Source: CAD feature listing. Evaluate the final solid. Frame: model axes, mm. A direction names the side the tool comes from. Round coordinates to 2 decimals unless told otherwise and drop trailing zeros. Loops run counter-clockwise (first coordinate to the right, second up) from the corner with the lowest first, then second, coordinate; pieces in that order, holes last. Notation, with made-up numbers: M 82.25,16.5 L 117.25,16.5 A23 ccw 117.25,34.5 Z; hole C -13.5,30 d4. An arc over 180 degrees is marked long. Write each question's results on one line, items separated by ' | '. Start each with the question number.
1. Set-up query: faces 1 (the flat face through (6, 2, -1)), 2 (the flat face through (11, 31, 0)), 3 (the flat face through (5, 18, -6.5)), 4 (the cylindrical face through (78.986, 8.474, -7.648)), 5 (the cylindrical face through (12.4, 25.27, 14.01)). Return all of +Z, -Z, +X, -X, +Y, -Y with unobstructed straight access to the full face (end or side cutting, diameter ignored); none if empty.
2. Section B-B on y = 18.5. Output: boundary loops of the cut face in (x, z), and give its area (3 significant figures).
3. Contact query for flat-ended pins moving along their axis: pin 1 Ø2 at (x, z) = (9.5, 0.5) entering from +Y; pin 2 Ø5 at (x, z) = (15, 0) entering from -Y; pin 3 Ø9 at (x, z) = (55.5, 0) entering from +Y; pin 4 Ø13 at (y, z) = (22, -2.5) entering from +X. Output: stop coordinate, or through.
4. Ray query, line 1 (Y direction, x = 3.75, z = 9); line 2 (Z direction, x = 8, y = 20.5); line 3 (Z direction, x = 12.5, y = 23.5). Return the intervals inside material, ascending.
5. Section D-D on z = 0. Give the number of separate pieces and of enclosed holes in the cut face, and give its area (3 significant figures).
6. Draft query along Z for faces 6 (the cylindrical face through (40.53, 0.57, 14.4)), 7 (the cylindrical face through (7, 32, 6)), 8 (the cylindrical face through (11.43, 34.4, 14.01)). Return one class per face: released by +Z, released by -Z, zero draft, split by the parting line, or undercut.
7. Section C-C on x = 44. Output: boundary loops of the cut face in (y, z).
8. Section A-A on x = 70. Output: boundary loops of the cut face in (y, z), and give its area (3 significant figures).
from build123d import *

# Parameters (mm, degrees)
BOSS_EXTRUDE1_DEPTH = 15
FILLET2_R           = 10
FILLET3_R           = 2
FILLET4_R           = 2
SHELL1_START        = 2
SHELL1_OUTLINE_W    = 33
SHELL1_OUTLINE_H    = 26
SHELL1_DEPTH        = 76
SKETCH2_R           = 2
CUT_EXTRUDE1_DEPTH  = 88.82938005
BOSS_EXTRUDE2_START = 6
SKETCH3_R           = 4
SKETCH3_R_2         = 2
BOSS_EXTRUDE2_DEPTH = 6
SKETCH4_W           = 26
SKETCH4_H           = 31
BOSS_EXTRUDE3_DEPTH = 10
SKETCH5_W           = 8
SKETCH5_H           = 8
CUT_EXTRUDE2_DEPTH  = 31
SKETCH6_W           = 8
SKETCH6_H           = 2
CUT_EXTRUDE3_DEPTH  = 6
FILLET5_R           = 5
FILLET6_R           = 2
SKETCH7_R           = 2
CUT_EXTRUDE4_DEPTH  = 89.600225733
CUT_EXTRUDE6_DEPTH  = 10


# Read off the part's stored shape, not the designer's step: Shell1
# Some blends are built 0.0001 mm under size
with BuildPart() as part:
    # Sketch1 → Boss-Extrude1 (new, symmetric)
    with BuildSketch(Plane.XY):
        with BuildLine():
            Line((0, 35), (0, 0))
            Line((0, 0), (80, 0))
            Line((80, 0), (80, 10))
            Line((80, 10), (60, 10))
            Line((60, 10), (13.403450014, 24.561421871))
            ThreePointArc((13.403450014, 24.561421871), (12.388618609, 25.28570887), (12, 26.470381827))
            Line((12, 26.470381827), (12, 33))
            ThreePointArc((12, 33), (11.414213562, 34.414213562), (10, 35))
            Line((10, 35), (0, 35))
        make_face()
    extrude(amount=BOSS_EXTRUDE1_DEPTH, both=True)

    # Fillet2
    fillet2_edges = [part.edges().sort_by_distance(p)[0] for p in [
        (60, 10, 0),
    ]]
    fillet(fillet2_edges, radius=FILLET2_R)

    # Fillet3
    fillet3_edges = [part.edges().sort_by_distance(p)[0] for p in [
        (80, 5, -15),
        (0, 17.5, -15),
        (80, 5, 15),
        (0, 17.5, 15),
    ]]
    fillet(fillet3_edges, radius=FILLET3_R)

    # Fillet4
    fillet4_edges = [part.edges().sort_by_distance(p)[0] for p in [
        (0, 0, 0),
        (40, 0, -15),
        (80, 0, 0),
        (40, 0, 15),
        (79.414213562, 0, 14.414213562),
        (79.414213562, 0, -14.414213562),
        (0.585786438, 0, 14.414213562),
        (0.585786438, 0, -14.414213562),
    ]]
    fillet(fillet4_edges, radius=FILLET4_R)

    # Shell1 outline → Shell1 (cut)
    with BuildSketch(Plane.YZ.offset(SHELL1_START)):
        with Locations((18.5, 0)):
            Rectangle(SHELL1_OUTLINE_W, SHELL1_OUTLINE_H)
    extrude(amount=SHELL1_DEPTH, mode=Mode.SUBTRACT)

    # Sketch2 → Cut-Extrude1 (cut, through all)
    with BuildSketch(Plane(origin=(0, 2, 0), x_dir=(1, 0, 0), z_dir=(0, 1, 0))):
        with Locations(Location((70, 0, 0), (0, 0, 270))):
            Circle(SKETCH2_R)
        with Locations(Location((55, 0, 0), (0, 0, 270))):
            Circle(SKETCH2_R)
        with Locations(Location((15, 0, 0), (0, 0, 270))):
            Circle(SKETCH2_R)
    extrude(amount=-CUT_EXTRUDE1_DEPTH, mode=Mode.SUBTRACT)

    # Sketch3 → Boss-Extrude2 (add)
    # profile 1 of 3: a face of its own
    with BuildSketch(Plane(origin=(0, 2, 0), x_dir=(1, 0, 0), z_dir=(0, 1, 0)).offset(BOSS_EXTRUDE2_START)):
        with Locations(Location((70, 0, 0), (0, 0, 270))):
            Circle(SKETCH3_R)
        with Locations(Location((70, 0, 0), (0, 0, 270))):
            Circle(SKETCH3_R_2, mode=Mode.SUBTRACT)
    # profile 2 of 3: a face of its own
    with BuildSketch(Plane(origin=(0, 2, 0), x_dir=(1, 0, 0), z_dir=(0, 1, 0)).offset(BOSS_EXTRUDE2_START)):
        with Locations(Location((55, 0, 0), (0, 0, 270))):
            Circle(SKETCH3_R)
        with Locations(Location((55, 0, 0), (0, 0, 270))):
            Circle(SKETCH3_R_2, mode=Mode.SUBTRACT)
    # profile 3 of 3: a face of its own
    with BuildSketch(Plane(origin=(0, 2, 0), x_dir=(1, 0, 0), z_dir=(0, 1, 0)).offset(BOSS_EXTRUDE2_START)):
        with Locations(Location((15, 0, 0), (0, 0, 270))):
            Circle(SKETCH3_R)
        with Locations(Location((15, 0, 0), (0, 0, 270))):
            Circle(SKETCH3_R_2, mode=Mode.SUBTRACT)
    extrude(amount=-BOSS_EXTRUDE2_DEPTH)

    # Sketch4 → Boss-Extrude3 (add)
    with BuildSketch(Plane(origin=(12, 0, 0), x_dir=(0, 0, -1), z_dir=(1, 0, 0))):
        with Locations((0, 17.5)):
            Rectangle(SKETCH4_W, SKETCH4_H)
    extrude(amount=-BOSS_EXTRUDE3_DEPTH)

    # Sketch5 → Cut-Extrude2 (cut)
    with BuildSketch(Plane(origin=(0, 33, 0), x_dir=(1, 0, 0), z_dir=(0, 1, 0))):
        with Locations((6, 0)):
            Rectangle(SKETCH5_W, SKETCH5_H)
    extrude(amount=-CUT_EXTRUDE2_DEPTH, mode=Mode.SUBTRACT)

    # Sketch6 → Cut-Extrude3 (cut)
    with BuildSketch(Plane.ZY.offset(-10)):
        with Locations((0, 32)):
            Rectangle(SKETCH6_W, SKETCH6_H)
    extrude(amount=-CUT_EXTRUDE3_DEPTH, mode=Mode.SUBTRACT)

    # Fillet5
    # the kernel refuses this fillet: 5 mm, written as the material it takes off along each edge
    with BuildSketch(Plane(origin=(24.5, 33, -4), x_dir=(0, 0, -1), z_dir=(-1, 0, 0))) as fillet5_piece_1_section:
        with BuildLine():
            CenterArc((FILLET5_R, FILLET5_R), FILLET5_R, 180, 90)
            Line((0, FILLET5_R), (0, 0))
            Line((0, 0), (FILLET5_R, 0))
        make_face()
    fillet5_piece_1 = extrude(amount=22.5, mode=Mode.PRIVATE)
    fillet5_piece_1 = split(fillet5_piece_1, bisect_by=Plane(origin=(11, 31, -5.295296425), z_dir=(0, 1, 0)), keep=Keep.TOP, mode=Mode.PRIVATE)
    add(fillet5_piece_1, mode=Mode.SUBTRACT)
    with BuildSketch(Plane(origin=(24.5, 33, -4), x_dir=(0, 0, -1), z_dir=(-1, 0, 0))) as fillet5_piece_2_section:
        with BuildLine():
            CenterArc((FILLET5_R, FILLET5_R), FILLET5_R, 180, 90)
            Line((0, FILLET5_R), (0, 0))
            Line((0, 0), (FILLET5_R, 0))
        make_face()
    fillet5_piece_2 = extrude(amount=22.5, mode=Mode.PRIVATE)
    fillet5_piece_2 = split(fillet5_piece_2, bisect_by=Plane(origin=(10, 30.265828048, -4.294049439), z_dir=(-1, 0, 0)), keep=Keep.TOP, mode=Mode.PRIVATE)
    add(fillet5_piece_2, mode=Mode.SUBTRACT)
    with BuildSketch(Plane(origin=(24.5, 33, 4), x_dir=(0, -1, 0), z_dir=(-1, 0, 0))) as fillet5_piece_3_section:
        with BuildLine():
            CenterArc((FILLET5_R, FILLET5_R), FILLET5_R, 180, 90)
            Line((0, FILLET5_R), (0, 0))
            Line((0, 0), (FILLET5_R, 0))
        make_face()
    fillet5_piece_3 = extrude(amount=22.5, mode=Mode.PRIVATE)
    fillet5_piece_3 = split(fillet5_piece_3, bisect_by=Plane(origin=(11, 31, 5.295296425), z_dir=(0, 1, 0)), keep=Keep.TOP, mode=Mode.PRIVATE)
    add(fillet5_piece_3, mode=Mode.SUBTRACT)
    with BuildSketch(Plane(origin=(24.5, 33, 4), x_dir=(0, -1, 0), z_dir=(-1, 0, 0))) as fillet5_piece_4_section:
        with BuildLine():
            CenterArc((FILLET5_R, FILLET5_R), FILLET5_R, 180, 90)
            Line((0, FILLET5_R), (0, 0))
            Line((0, 0), (FILLET5_R, 0))
        make_face()
    fillet5_piece_4 = extrude(amount=22.5, mode=Mode.PRIVATE)
    fillet5_piece_4 = split(fillet5_piece_4, bisect_by=Plane(origin=(10, 30.265828048, 4.294049439), z_dir=(-1, 0, 0)), keep=Keep.TOP, mode=Mode.PRIVATE)
    add(fillet5_piece_4, mode=Mode.SUBTRACT)

    # Fillet6
    fillet6_edges = [part.edges().sort_by_distance(p)[0] for p in [
        (2, 33, -11),
        (2, 31.535533906, -5.464466094),
        (10, 29.58113883, -4.25658351),
        (2, 33, 11),
        (2, 31.535533906, 5.464466094),
        (2, 15, -4),
        (10, 15, -4),
        (2, 15, 4),
        (10, 29.58113883, 4.25658351),
        (6, 2, 4),
        (10, 15, 4),
    ]]
    fillet(fillet6_edges, radius=FILLET6_R - 0.0001)  # a hair under: the kernel refuses the full size

    # Sketch7 → Cut-Extrude4 (cut, through all)
    with BuildSketch(Plane.ZY):
        with Locations(Location((-9, 29, 0), (0, 0, 270))):
            Circle(SKETCH7_R)
        with Locations(Location((-9, 7, 0), (0, 0, 270))):
            Circle(SKETCH7_R)
        with Locations((9, 7)):
            Circle(SKETCH7_R)
        with Locations((9, 29)):
            Circle(SKETCH7_R)
    extrude(amount=-CUT_EXTRUDE4_DEPTH, mode=Mode.SUBTRACT)

    # Sketch8 → Cut-Extrude6 (cut)
    with BuildSketch(Plane.ZY):
        with BuildLine():
            Line((-11.5, 13), (-11.5, 23))
            ThreePointArc((-11.5, 23), (-9, 25.5), (-6.5, 23))
            Line((-6.5, 23), (-6.5, 13))
            ThreePointArc((-6.5, 13), (-9, 10.5), (-11.5, 13))
        make_face()
        with BuildLine():
            Line((11.5, 13), (11.5, 23))
            ThreePointArc((11.5, 23), (9, 25.5), (6.5, 23))
            Line((6.5, 23), (6.5, 13))
            ThreePointArc((6.5, 13), (9, 10.5), (11.5, 13))
        make_face()
    extrude(amount=-CUT_EXTRUDE6_DEPTH, mode=Mode.SUBTRACT)


solid = part.part
Taken from the geometry:
1) face 1: +Y | face 2: +X, +Y | face 3: -X | face 4: +X, -X | face 5: +Z, -Z, +X, +Y
2) outline: M 0,-13 A2 ccw 2,-15 L 32.8,-15 L 32.8,-13 L 12,-13 L 12,13 L 32.8,13 L 32.8,15 L 2,15 A2 ccw 0,13 L 0,11.5 L 10,11.5 L 10,6.5 L 0,6.5 L 0,-6.5 L 10,-6.5 L 10,-11.5 L 0,-11.5 Z; hole M 2,-2 A2 ccw 4,-4 L 8,-4 A2 ccw 10,-2 L 10,2 A2 ccw 8,4 L 4,4 A2 ccw 2,2 Z | area: 281 mm^2
3) pin 1: y = 31 | pin 2: y = 0 | pin 3: y = 8 | pin 4: x = 12
4) line 1: 0 to 5, 9 to 10.5, 25.5 to 27, 31 to 33.02 | line 2: -15 to -11.5, -6.5 to -4, 4 to 6.5, 11.5 to 15 | line 3: -15 to -13, 13 to 15
5) separate pieces: 4 | enclosed holes: 0 | area: 340 mm^2
6) face 6: released by +Z | face 7: undercut | face 8: zero draft
7) outline: M 0,-13 A2 ccw 2,-15 L 15,-15 L 15,-13 L 2,-13 L 2,13 L 15,13 L 15,15 L 2,15 A2 ccw 0,13 Z
8) outline: M 0,-13 A2 ccw 2,-15 L 10,-15 L 10,-13 L 2,-13 L 2,-4 L 8,-4 L 8,-2 L 0,-2 Z; M 0,2 L 8,2 L 8,4 L 2,4 L 2,13 L 10,13 L 10,15 L 2,15 A2 ccw 0,13 Z | area: 106 mm^2
